from build123d import *

# Parameters (mm, degrees)
CROQUIS1_W              = 45
CROQUIS1_H              = 45
SALIENTE_EXTRUIR1_DEPTH = 300
CROQUIS4_W              = 18
CROQUIS4_H              = 34
CORTAR_EXTRUIR2_DEPTH   = 46
CROQUIS8_W              = 35
CROQUIS8_H              = 35
CORTAR_EXTRUIR3_DEPTH   = 301
CROQUIS9_W              = 35
CROQUIS9_H              = 21.174410022
CORTAR_EXTRUIR4_DEPTH   = 10
CROQUIS10_R             = 1
CORTAR_EXTRUIR5_DEPTH   = 10
CROQUIS11_W             = 45
CROQUIS11_H             = 26.387879272
CORTAR_EXTRUIR6_DEPTH   = 46


with BuildPart() as part:
    # Croquis1 → Saliente-Extruir1 (new body)
    with BuildSketch(Plane(origin=(0, 0, 0), x_dir=(1, 0, 0), z_dir=(0, 1, 0))):
        Rectangle(CROQUIS1_W, CROQUIS1_H)
    extrude(amount=SALIENTE_EXTRUIR1_DEPTH)

    # Croquis4 → Cortar-Extruir2 (cut, through all)
    with BuildSketch(Plane.ZY.offset(22.5)):
        with Locations((13.5, 17)):
            Rectangle(CROQUIS4_W, CROQUIS4_H)
    extrude(amount=-CORTAR_EXTRUIR2_DEPTH, mode=Mode.SUBTRACT)

    # Croquis8 → Cortar-Extruir3 (cut, through all)
    with BuildSketch(Plane(origin=(0, 300, 0), x_dir=(1, 0, 0), z_dir=(0, 1, 0))):
        Rectangle(CROQUIS8_W, CROQUIS8_H)
    extrude(amount=-CORTAR_EXTRUIR3_DEPTH, mode=Mode.SUBTRACT)

    # Croquis9 → Cortar-Extruir4 (cut)
    with BuildSketch(Plane(origin=(0, 0, -22.5), x_dir=(-1, 0, 0), z_dir=(0, 0, -1))):
        with Locations((0, 260)):
            Rectangle(CROQUIS9_W, CROQUIS9_H)
    extrude(amount=-CORTAR_EXTRUIR4_DEPTH, mode=Mode.SUBTRACT)

    # Croquis10 → Cortar-Extruir5 (cut)
    with BuildSketch(Plane.XY.offset(22.5)):
        with Locations((0, 260)):
            Circle(CROQUIS10_R)
    extrude(amount=-CORTAR_EXTRUIR5_DEPTH, mode=Mode.SUBTRACT)

    # Croquis11 → Cortar-Extruir6 (cut, through all)
    with BuildSketch(Plane.XY.offset(22.5)):
        with Locations((0, 286.806060364)):
            Rectangle(CROQUIS11_W, CROQUIS11_H)
    extrude(amount=-CORTAR_EXTRUIR6_DEPTH, mode=Mode.SUBTRACT)


solid = part.part
Could you check a few things on this model? Use its own coordinates, in mm. A direction names the side the tool comes from. Coordinates: 2 decimals unless noted, no trailing zeros. Write each loop counter-clockwise with the first axis right and the second up, starting at its lowest first coordinate (ties: lowest second). Pieces come first, ordered by that corner, then holes. Notation, with made-up numbers: (89, -33.75) - (145, -33.75) arc R8 ccw to (145, -28.75) - close; hole circle Ø9 at (-37.5, -23). An arc over 180 degrees is marked (long way). Put each result on its own line as item: value. Start each with the question number.
Q1. Please list where these lines run through material, in increasing order: L1, parallel to Y at x = 0, z = 21.15; L2, parallel to X at y = 146, z = 0.5; L3, parallel to X at y = 260, z = 20.
Q2. Thinking about a two-plate mould opening in X: for faces 1 (the flat face through (0, 270.587, -20)), 2 (the flat face through (0, 135, -22.5)), 3 (the flat face through (22.5, 135, 0)), 4 (the flat face through (0, 249.413, -20)), which applies, pulls with the +X half, pulls with the -X half, needs draft (parallel to the pull), parting line crosses it, or undercut?
Q3. I want a section at A-A on x = 14.5. Write out the boundary of the cut face in (y, z).
Q4. I want a section at C-C on y = 78.5. Write out the boundary of the cut face in (x, z).
Q5. I want a section at B-B on z = -2.5. Write out the boundary of the cut face in (x, y), plus the area to 3 significant figures.
Q6. Which directions (+Z, -Z, +X, -X, +Y, -Y) give clear straight access to the entire face, cutting with the end or side of a thin tool? Please do faces 5 (the flat face through (0, 34, 19)), 6 (the flat face through (0, 126, -17.5)), 7 (the flat face through (0, 0, -18)).
Q7. I'm going to push flat-ended pins straight in: P1, Ø3, axis at x = 9, z = 18, coming from the -Y side; P2, Ø2.5, axis at x = 0, y = 260, coming from the -Z side; P3, Ø5.5, axis at x = -21, y = 24, coming from the +Z side. Where does each tip first touch, or does it pass through?
Checks:
1. L1: 34 to 259, 261 to 273.61
1. L2: -22.5 to -17.5, 17.5 to 22.5
1. L3: -22.5 to -1, 1 to 22.5
2. face 1: undercut
2. face 2: needs draft
2. face 3: pulls with the +X half
2. face 4: undercut
3. outline: (0, -22.5) - (249.41, -22.5) - (249.41, -17.5) - (0, -17.5) - close; (34, 17.5) - (273.61, 17.5) - (273.61, 22.5) - (34, 22.5) - close; (270.59, -22.5) - (273.61, -22.5) - (273.61, -17.5) - (270.59, -17.5) - close
4. outline: (-22.5, -22.5) - (22.5, -22.5) - (22.5, 22.5) - (-22.5, 22.5) - close; hole (-17.5, -17.5) - (17.5, -17.5) - (17.5, 17.5) - (-17.5, 17.5) - close
5. outline: (-22.5, 0) - (-17.5, 0) - (-17.5, 273.61) - (-22.5, 273.61) - close; (17.5, 0) - (22.5, 0) - (22.5, 273.61) - (17.5, 273.61) - close
5. area: 2,740 mm²
6. face 5: +Z, +X, -X, -Y
6. face 6: +Y, -Y
6. face 7: +Z, -Z, +X, -X, -Y
7. P1: y = 34
7. P2: z = 17.5
7. P3: z = 4.5
